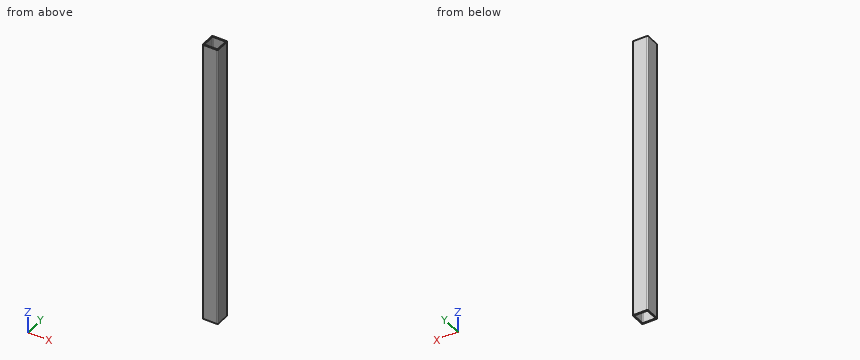
from build123d import *

# Parameters (mm, degrees)
BOSS_EXTRUDE1_DEPTH = 737
SKETCH2_W           = 38.1
SKETCH2_H           = 25.1
CUT_EXTRUDE1_DEPTH  = 739.966995203


with BuildPart() as part:
    # Sketch1 → Boss-Extrude1 (new body)
    with BuildSketch(Plane.XY):
        with BuildLine():
            Line((2.54, 0), (35.56, 0))
            ThreePointArc((35.56, 0), (37.356051224, -0.743948776), (38.1, -2.54))
            Line((38.1, -2.54), (38.1, -35.56))
            ThreePointArc((38.1, -35.56), (37.356051224, -37.356051224), (35.56, -38.1))
            Line((35.56, -38.1), (2.54, -38.1))
            ThreePointArc((2.54, -38.1), (0.743948776, -37.356051224), (0, -35.56))
            Line((0, -35.56), (0, -2.54))
            ThreePointArc((0, -2.54), (0.743948776, -0.743948776), (2.54, 0))
        make_face()
        with BuildLine():
            Line((5.3086, -2.7686), (32.7914, -2.7686))
            ThreePointArc((32.7914, -2.7686), (34.587451224, -3.512548776), (35.3314, -5.3086))
            Line((35.3314, -5.3086), (35.3314, -32.7914))
            ThreePointArc((35.3314, -32.7914), (34.587451224, -34.587451224), (32.7914, -35.3314))
            Line((32.7914, -35.3314), (5.3086, -35.3314))
            ThreePointArc((5.3086, -35.3314), (3.512548776, -34.587451224), (2.7686, -32.7914))
            Line((2.7686, -32.7914), (2.7686, -5.3086))
            ThreePointArc((2.7686, -5.3086), (3.512548776, -3.512548776), (5.3086, -2.7686))
        make_face(mode=Mode.SUBTRACT)
    extrude(amount=BOSS_EXTRUDE1_DEPTH)

    # Sketch2 → Cut-Extrude1 (cut, through all)
    with BuildSketch(Plane(origin=(0, 0, 0), x_dir=(1, 0, 0), z_dir=(0, 1, 0))):
        with Locations((19.05, -724.45)):
            Rectangle(SKETCH2_W, SKETCH2_H)
    extrude(amount=-CUT_EXTRUDE1_DEPTH, mode=Mode.SUBTRACT)


solid = part.part
Work out the finished part from the listing and answer in its coordinate system (mm). Round coordinates to 2 decimals unless told otherwise and drop trailing zeros. Loops run counter-clockwise (first coordinate to the right, second up) from the corner with the lowest first, then second, coordinate; pieces in that order, holes last. Notation, with made-up numbers: M -28.75,65 L 15.25,65 A37 ccw 15.25,104 Z; hole C 7.5,-38.5 d4. An arc over 180 degrees is marked long. One line per question, with ' | ' between items. Start each with the question number.
(1) Find the intervals of material crossed by line 1 (X direction, y = -26, z = 294); line 2 (Y direction, x = 28.5, z = 147); line 3 (X direction, y = -33.5, z = 399.5), in increasing order.
(2) A flat-ended cylindrical pin translates along its axis: pin 1 Ø1 at (x, y) = (26.5, -34) entering from -Z (3 decimals). Find the tip coordinate at first contact, or state that the pin passes through.
(3) A cutting plane is placed at B-B on y = -15. Write down the section's boundary in (x, z), plus the area to 3 significant figures.
(4) A cutting plane is placed at A-A on x = 24.5. Write down the section's boundary in (y, z), plus the area to 3 significant figures.
(5) A cutting plane is placed at C-C on z = 167. Write down the section's boundary in (x, y).
Geometry check:
1) line 1: x = 0 to 2.77, 35.33 to 38.1 | line 2: y = -38.1 to -35.33, -2.77 to 0 | line 3: x = 0 to 2.87, 35.23 to 38.1
2) pin 1: passes through
3) outline: M 0,0 L 2.77,0 L 2.77,711.9 L 0,711.9 Z; M 35.33,0 L 38.1,0 L 38.1,711.9 L 35.33,711.9 Z | area: 3,940 mm²
4) outline: M -38.1,0 L -35.33,0 L -35.33,711.9 L -38.1,711.9 Z; M -2.77,0 L 0,0 L 0,711.9 L -2.77,711.9 Z | area: 3,940 mm²
5) outline: M 0,-35.56 A2.54 ccw 2.54,-38.1 L 35.56,-38.1 A2.54 ccw 38.1,-35.56 L 38.1,-2.54 A2.54 ccw 35.56,0 L 2.54,0 A2.54 ccw 0,-2.54 Z; hole M 2.77,-32.79 A2.54 ccw 5.31,-35.33 L 32.79,-35.33 A2.54 ccw 35.33,-32.79 L 35.33,-5.31 A2.54 ccw 32.79,-2.77 L 5.31,-2.77 A2.54 ccw 2.77,-5.31 Z
